from build123d import *

# Parameters (mm, degrees)
F1_DEPTH = 25.4


with BuildPart() as f1:
    # F0 (on Front) → F1 (new body)
    with BuildSketch(Plane.XZ):
        Polygon((25.4, -25.4), (25.4, 25.4), (-25.4, 25.4), (-25.4, -25.4), (0, -25.4), (0, -6.536582), (10.239619, -6.536582), (10.239619, -16.214322), (10.239619, -25.4), align=None)
        Polygon((-13.493889, 7.98003), (-17.180648, 7.98003), (-17.180648, 14.547069), (-17.180648, 21.114107), (-13.493889, 21.114107), (-9.807131, 21.114107), (-9.807131, 14.547069), (-9.807131, 7.98003), align=None, mode=Mode.SUBTRACT)
        Polygon((13.46553, 7.05834), (9.548349, 7.05834), (9.548349, 14.086224), (9.548349, 21.114107), (13.46553, 21.114107), (17.382711, 21.114107), (17.382711, 14.086224), (17.382711, 7.05834), align=None, mode=Mode.SUBTRACT)
        Polygon((-25.4, 25.4), (25.4, 25.4), (0, 45.190681), align=None)
    extrude(amount=F1_DEPTH)


solid = f1.part
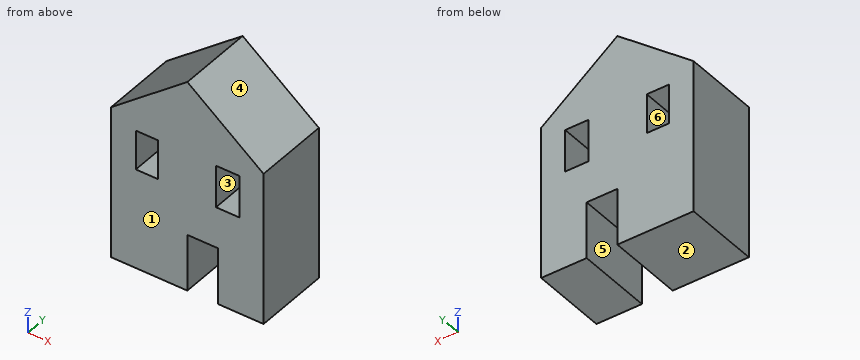
The listing builds one solid part. Answer for the finished solid, in the listing's coordinates (mm). Face numbers are marked on the shaded views. A direction names the side the tool comes from. Give positions to 0.01 mm unless a question says otherwise; leave off trailing zeros. Write each loop counter-clockwise with the first axis right and the second up, starting at its lowest first coordinate (ties: lowest second). Pieces come first, ordered by that corner, then holes.
Item 1: Flat-ended cylindrical pins translate along their axes: P1, Ø2.5, axis at x = 13, y = -12.5, coming from the +Z side; P2, Ø3, axis at x = 16.5, y = -5, coming from the +Z side; P3, Ø2, axis at x = 5, y = -17.5, coming from the +Z side. Find the tip coordinate at first contact, or state that the pin passes through.
Item 2: Section D-D, the plane x = -16 is taken. Write down the section's boundary in (y, z).
Item 3: Section A-A, the plane y = -16.5 is taken. Write down the section's boundary in (x, z).
Item 4: Which of the six approach directions +Z, -Z, +X, -X, +Y, -Y give full straight-line access (tool end or side, diameter ignored) to the marked faces 4, 5 and 6?
Item 5: Section C-C, the plane z = -8 is taken. Write down the section's boundary in (x, y), plus the area to 3 significant figures.
Item 6: Determine the mould class of the marked faces 1, 2 and 3 for opening direction Z: released by +Z, released by -Z, zero draft, split by the parting line, or undercut.
Item 7: Section B-B, the plane z = 15.5 is taken. Write down the section's boundary in (x, y), plus the area to 3 significant figures.
Item 8: Find the intervals of material crossed by line 1 along X through (y, z) = (-17.25, 9.5); line 2 along X through (y, z) = (-13.25, -18); line 3 along Z through (x, y) = (-13, -16.75), in increasing order.
Completed:
1. P1: stops at z = 36.04
1. P2: stops at z = 33.5
1. P3: stops at z = 42.07
2. outline: (-25.4, -25.4) - (0, -25.4) - (0, 7.98) - (-25.4, 7.98) - close; (-25.4, 21.11) - (0, 21.11) - (0, 32.72) - (-25.4, 32.72) - close
3. outline: (-25.4, -25.4) - (0, -25.4) - (0, -6.54) - (10.24, -6.54) - (10.24, -25.4) - (25.4, -25.4) - (25.4, 25.4) - (0, 45.19) - (-25.4, 25.4) - close; hole (-17.18, 7.98) - (-9.81, 7.98) - (-9.81, 21.11) - (-17.18, 21.11) - close; hole (9.55, 7.06) - (17.38, 7.06) - (17.38, 21.11) - (9.55, 21.11) - close
4. face 4: +Z, +X, +Y, -Y
4. face 5: -Z, +Y, -Y
4. face 6: +Y, -Y
5. outline: (-25.4, -25.4) - (0, -25.4) - (0, 0) - (-25.4, 0) - close; (10.24, -25.4) - (25.4, -25.4) - (25.4, 0) - (10.24, 0) - close
5. area: 1,030 mm2
6. face 1: zero draft
6. face 2: released by -Z
6. face 3: undercut
7. outline: (-25.4, -25.4) - (-17.18, -25.4) - (-17.18, 0) - (-25.4, 0) - close; (-9.81, -25.4) - (9.55, -25.4) - (9.55, 0) - (-9.81, 0) - close; (17.38, -25.4) - (25.4, -25.4) - (25.4, 0) - (17.38, 0) - close
7. area: 904 mm2
8. line 1: x = -25.4 to -17.18, -9.81 to 9.55, 17.38 to 25.4
8. line 2: x = -25.4 to 0, 10.24 to 25.4
8. line 3: z = -25.4 to 7.98, 21.11 to 35.06
